```python
from build123d import *

# Parameters (mm, degrees)
SKETCH1_R               = 37.5
SKETCH1_R_2             = 34
BOSS_EXTRUDE1_DEPTH     = 10
BOSS_EXTRUDE2_DEPTH     = 37.2
SKETCH2_3_R             = 37.5
SKETCH2_3_R_2           = 34
BOSS_EXTRUDE3_DEPTH     = 94.7
CUT_EXTRUDE2_DEPTH      = 60
CUT_EXTRUDE2_DEPTH_BACK = 60
SKETCH3_R               = 50
SKETCH4_R               = 22.6
SKETCH4_R_2             = 19.6
BOSS_EXTRUDE4_DEPTH     = 40
FILLET1_R               = 5


with BuildPart() as part:
    # Sketch1 → Boss-Extrude1 (new body)
    # profile 1 of 2: a face of its own
    with BuildSketch(Plane(origin=(0, 0, 0), x_dir=(1, 0, 0), z_dir=(0, 1, 0))):
        with Locations(Location((0, 0, 0), (0, 0, 270))):
            Circle(SKETCH1_R)
        Circle(SKETCH1_R_2, mode=Mode.SUBTRACT)
    # profile 2 of 2: a face of its own
    with BuildSketch(Plane(origin=(0, 0, 0), x_dir=(1, 0, 0), z_dir=(0, 1, 0))):
        Circle(SKETCH1_R_2)
    extrude(amount=BOSS_EXTRUDE1_DEPTH)

    # Sketch2 → Boss-Extrude2 (add)
    with BuildSketch(Plane(origin=(0, 10, 0), x_dir=(1, 0, 0), z_dir=(0, 1, 0))):
        with BuildLine():
            ThreePointArc((25.708704752, 22.25), (0, 34), (-25.708704752, 22.25))
            Line((-25.708704752, 22.25), (-10, 22.25))
            Line((-10, 22.25), (-10, 32.25))
            Line((-10, 32.25), (10, 32.25))
            Line((10, 32.25), (10, 22.25))
            Line((10, 22.25), (25.708704752, 22.25))
        make_face()
        with BuildLine():
            Line((-10, -3), (-33.867388444, -3))
            ThreePointArc((-33.867388444, -3), (-33.022694549, -8.09330864), (-31.416556145, -13))
            Line((-31.416556145, -13), (31.416556145, -13))
            ThreePointArc((31.416556145, -13), (33.022694549, -8.09330864), (33.867388444, -3))
            Line((33.867388444, -3), (10, -3))
            Line((10, -3), (10, -8))
            Line((10, -8), (-10, -8))
            Line((-10, -8), (-10, -3))
        make_face()
    extrude(amount=BOSS_EXTRUDE2_DEPTH)

    # Sketch2_3 → Boss-Extrude3 (add)
    with BuildSketch(Plane(origin=(0, 10, 0), x_dir=(1, 0, 0), z_dir=(0, 1, 0))):
        with Locations(Location((0, 0, 0), (0, 0, 270))):
            Circle(SKETCH2_3_R)
        with Locations(Location((0, 0, 0), (0, 0, 139.124938123))):
            Circle(SKETCH2_3_R_2, mode=Mode.SUBTRACT)
    extrude(amount=BOSS_EXTRUDE3_DEPTH)

    # Sketch3 → Cut-Extrude2 (cut, two sides: drawn at the far end of the back side and taken through both)
    with BuildSketch(Plane.XY.offset(-CUT_EXTRUDE2_DEPTH_BACK)):
        with Locations((0, 104.7)):
            Circle(SKETCH3_R)
    extrude(amount=CUT_EXTRUDE2_DEPTH + CUT_EXTRUDE2_DEPTH_BACK, mode=Mode.SUBTRACT)

    # Sketch4 → Boss-Extrude4 (add)
    with BuildSketch(Plane.XZ):
        with Locations(Location((0, 0, 0), (0, 0, 90))):
            Circle(SKETCH4_R)
        with Locations(Location((0, 0, 0), (0, 0, 270))):
            Circle(SKETCH4_R_2, mode=Mode.SUBTRACT)
    extrude(amount=BOSS_EXTRUDE4_DEPTH)

    # Fillet1
    fillet1_edges = [part.edges().sort_by_distance(p)[0] for p in [
        (0, 0, -37.5),
    ]]
    fillet(fillet1_edges, radius=FILLET1_R)


solid = part.part
```
Here's how the part is built. I have some questions about the finished solid (model axes, mm). A direction names the side the tool comes from. Round coordinates to 2 decimals unless told otherwise and drop trailing zeros. Order: outer loops, then holes, each group sorted by start corner. A loop starts at its lowest first (then second) coordinate and runs counter-clockwise, first axis right, second up. Notation, with made-up numbers: M -27,60.25 L -13,60.25 A8 ccw -13,73.25 Z; hole C 51.5,80.25 d10. An arc over 180 degrees is marked long. One line per question, with ' | ' between items.
1) For faces 1 (the face through (15.3, 57.1, -30.7)), 2 (the face through (7, 0, -22)), 3 (the face through (10, 28, 5)), which set-ups out of +Z, -Z, +X, -X, +Y, -Y let a thin tool reach every point of the face, with its end or its side?
Working result:
face 1: +Z, -Z, +Y | face 2: -Y | face 3: +Y
2) For pin 1 Ø2 at (x, y) = (-5, 25.5) entering from -Z; pin 2 Ø10 at (x, z) = (24.5, 19.5) entering from +Y; pin 3 Ø6 at (y, z) = (51, 12) entering from -X, each with a flat end and sliding along its axis, tell me the tip position at first contact or that it passes through.
Working result:
pin 1: z = -37.29 | pin 2: y = 64.33 | pin 3: x = -36.4
3) If we mould it in two halves opening along Z, with no side actions, what happens to faces 4 (the face through (13.8, -19.7, -17.9)), 5 (the face through (-19, -40, -7)), 6 (the face through (0, 47.2, 9))? For each: +Z half, -Z half, draft (parallel to the pull), parting line (faces both ways), or undercut.
Working result:
face 4: parting line | face 5: draft | face 6: undercut
4) I want a section at A-A, the plane z = 0. Write out the boundary of the cut face in (x, y).
Working result:
outline: M -37.5,5 A5 ccw -32.5,0 L -22.6,0 L -22.6,-40 L -19.6,-40 L -19.6,0 L 19.6,0 L 19.6,-40 L 22.6,-40 L 22.6,0 L 32.5,0 A5 ccw 37.5,5 L 37.5,71.63 A50 cw 34,68.04 L 34,10 L -34,10 L -34,68.04 A50 cw -37.5,71.63 Z
5) I want a section at B-B, the plane y = 56.5. Write out the boundary of the cut face in (x, z), then the cut area to 3 significant figures.
Working result:
outline: M -13.3,-35.06 L -13.3,-31.29 A34 cw -13.3,31.29 L -13.3,35.06 A37.5 ccw Z; M 13.3,-35.06 A37.5 ccw 13.3,35.06 L 13.3,31.29 A34 cw 13.3,-31.29 Z | area: 595 mm²
6) I want a section at D-D, the plane x = 0. Write out the boundary of the cut face in (y, z).
Working result:
outline: M -40,-22.6 L 0,-22.6 L 0,-32.5 A5 ccw 5,-37.5 L 54.7,-37.5 L 54.7,-34 L 47.2,-34 L 47.2,-32.25 L 10,-32.25 L 10,8 L 47.2,8 L 47.2,13 L 10,13 L 10,34 L 54.7,34 L 54.7,37.5 L 5,37.5 A5 ccw 0,32.5 L 0,22.6 L -40,22.6 L -40,19.6 L 0,19.6 L 0,-19.6 L -40,-19.6 Z
7) I want a section at C-C, the plane y = 38. Write out the boundary of the cut face in (x, z), then the cut area to 3 significant figures.
Working result:
outline: C 0,0 d75; hole M -33.87,3 A34 ccw -25.71,-22.25 L -10,-22.25 L -10,-32.25 L 10,-32.25 L 10,-22.25 L 25.71,-22.25 A34 ccw 33.87,3 L 10,3 L 10,8 L -10,8 L -10,3 Z; hole M -31.42,13 L 31.42,13 A34 ccw Z | area: 1,560 mm²
8) I need wall thicknesses on line 1 along Z through (x, y) = (0, 31); line 2 along X through (y, z) = (24, 0). Which ranges of each line are inside material? Lowest first, please.
Working result:
line 1: -37.5 to -32.25, 8 to 13, 34 to 37.5 | line 2: -37.5 to -34, 34 to 37.5
